Autodesk Inventor part; units mm, degrees
ref_plane "YZ Plane" through (0, 0, 0) normal (1, 0, 0) x (0, 1, 0)
ref_plane "XZ Plane" through (0, 0, 0) normal (0, 1, 0) x (-1, 0, 0)
ref_plane "XY Plane" through (0, 0, 0) normal (0, 0, 1) x (1, 0, 0)
sketch "Sketch1" plane through (0, 0, 0) normal (0, 0, 1) x (1, 0, 0)
  line L0 (0, 0) -> (52.5, 0)
  line L1 (63.5, 0) -> (63.5, 1.5)
  line L2 (0, 1.5) -> (0, 0)
  arc A0 (63.5, 1.5) -> (50.5, 1.5) centre (57, -3.9686) ccw
  arc A1 (61.5, 0) -> (52.5, 0) centre (57, -3.9686) ccw
  line L3 (61.5, 0) -> (63.5, 0)
  line L4 (52.5, 0) -> (61.5, 0) construction
  line L5 (59.4686, 1.5) -> (54.5314, 1.5) construction
  line L6 (54.5314, 1.5) -> (50.5, 1.5) construction
  line L7 (50.5, 1.5) -> (0, 1.5)
  line L8 (63.5, 1.5) -> (59.4686, 1.5) construction
  dimension "d0" = 63.5
  dimension "d1" = 1.5
  dimension "d3" = 9
  dimension "d4" = 6
  dimension "d5" = 2
extrude "Extrusion1" add sketch "Sketch1" along normal blind 15
sketch "Sketch2" plane through (0, 1.5, 0) normal (0, 1, 0) x (1, 0, 0)
  line L0 (50.5, 0) -> (0, 0)
  line L1 (0, 0) -> (0, -15)
  line L2 (50.5, -15) -> (0, -15)
  line L3 (3.38, 0) -> (3.38, -15) construction
  line L4 (3.38, -7.5) -> (15.38, -7.5) construction
  dimension "d9" = 3.38
  dimension "d10" = 12
hole "Hole1" at (3.38, 1.5, 7.5) at (15.38, 1.5, 7.5) direction (0, -1, 0) diameter 2 end through all
fillet "Fillet1" radius 1 3 edges at (63.5, 0, 7.5) (63.5, 1.5, 7.5) (61.5, 0, 7.5)
fillet "Fillet2" radius 5 1 edges at (50.5, 1.5, 7.5)
sketch "Sketch3" plane through (0, 0, 0) normal (0, -1, 0) x (1, 0, 0)
  line L0 (0, 15) -> (52.5, 15)
  line L1 (0, 0) -> (0, 15)
  line L2 (25, 20.9607) -> (67.8053, 20.9607)
  line L3 (67.8053, 20.9607) -> (67.8053, 10)
  line L4 (67.8053, 10) -> (25, 10)
  line L5 (25, 10) -> (25, 20.9607)
  dimension "d20" = 5
  dimension "d21" = 25
extrude "Extrusion2" cut sketch "Sketch3" against normal blind 8
fillet "Fillet3" radius 2 4 edges at (25, 0.75, 15) (25, 0.75, 10) (0, 0.75, 15) (0, 0.75, 0)
properties part number "hand2"
Verification items for the finished model (mm, model axes). A direction names the side the tool comes from. Round coordinates to 2 decimals unless told otherwise and drop trailing zeros. Loops run counter-clockwise (first coordinate to the right, second up) from the corner with the lowest first, then second, coordinate; pieces in that order, holes last. Notation, with made-up numbers: (67, 35) - (72, 35) arc R23 ccw to (72, 56) - close; hole circle Ø4 at (-4.5, 33). An arc over 180 degrees is marked (long way). Answer in a Markdown table with one row per item. Add a question column.
Q1. Section check D-D on x = 11. Enter the section's corners in (y, z).
Q2. Tool access check on faces 1 (the face through (50, 1, 10)), 2 (the face through (63.199, 0.285, 5.07)), 3 (the face through (25, 1.5, 6)). Record the directions out of +Z, -Z, +X, -X, +Y, -Y that give a thin tool (end or side, any length) a straight path to the whole face; none if there is none.
Q3. Section check C-C on z = 4.25. Enter the section's corners in (x, y).
Q4. Section check B-B on z = 7.5. Enter the section's corners in (x, y).
Q5. Gauge pin test, flat ends, axial feed: pin 1 (0.8 mm diameter, centred on y = 1, z = 12.5, fed in from +X); pin 2 (1.4 mm diameter, centred on x = 52, y = 3, fed in from +Z); pin 3 (6 mm diameter, centred on x = 21.5, z = 7.5, fed in from +Y); pin 4 (1 mm diameter, centred on x = 45.5, z = 2.5, fed in from -Y). Record the tip position at first contact, or that the pin passes through.
Q6. Material ranges on line 1 (Z direction, x = 15.38, y = 0.85); line 2 (X direction, y = 0.5, z = 7.5); line 3 (Y direction, x = 21.5, z = 8.5), recorded low to high.
Q7. Release check for a two-part mould opening along Z. For faces 4 (the face through (57.51, 4.51, 4.93)), 5 (the face through (3.34, 0.74, 6.5)), 6 (the face through (0.6, 0.74, 14.43)) record: pulls with the +Z half, pulls with the -Z half, needs draft (parallel to the pull), parting line crosses it, or undercut.
Q8. Section check A-A on x = 3.38. Enter the section's corners in (y, z).
Found:
| question | item | result |
|---|---|---|
| 1 | outline | (0, 0) - (1.5, 0) - (1.5, 15) - (0, 15) - close |
| 2 | face 1 | +Z, +X, +Y, -Y |
| 2 | face 2 | +Z, -Z, +X, -Y |
| 2 | face 3 | +Z, -Z, -X, +Y |
| 3 | outline | (0, 0) - (52.5, 0) arc R6 cw to (61.23, 0.29) arc R1 ccw to (61.93, 0) - (62.5, 0) arc R1 ccw to (63.5, 1) - (63.5, 1.12) arc R1 ccw to (63.23, 1.8) arc R8.49 ccw to (51.64, 2.62) arc R5 cw to (48.48, 1.5) - (0, 1.5) - close |
| 4 | outline | (0, 0) - (2.38, 0) - (2.38, 1.5) - (0, 1.5) - close; (4.38, 0) - (14.38, 0) - (14.38, 1.5) - (4.38, 1.5) - close; (16.38, 0) - (52.5, 0) arc R6 cw to (61.23, 0.29) arc R1 ccw to (61.93, 0) - (62.5, 0) arc R1 ccw to (63.5, 1) - (63.5, 1.12) arc R1 ccw to (63.23, 1.8) arc R8.49 ccw to (51.64, 2.62) arc R5 cw to (48.48, 1.5) - (16.38, 1.5) - close |
| 5 | pin 1 | stops at x = 25 |
| 5 | pin 2 | stops at z = 10 |
| 5 | pin 3 | stops at y = 1.5 |
| 5 | pin 4 | stops at y = 0 |
| 6 | line 1 | z = 0 to 6.5, 8.5 to 15 |
| 6 | line 2 | x = 0 to 2.38, 4.38 to 14.38, 16.38 to 53, 61 to 63.37 |
| 6 | line 3 | y = 0 to 1.5 |
| 7 | face 4 | needs draft |
| 7 | face 5 | undercut |
| 7 | face 6 | pulls with the +Z half |
| 8 | outline | (0, 0) - (1.5, 0) - (1.5, 6.5) - (0, 6.5) - close; (0, 8.5) - (1.5, 8.5) - (1.5, 15) - (0, 15) - close |
